from build123d import *

# Parameters (mm, degrees)
SKETCH001_W = 2773.187988
SKETCH001_H = 2729.466553
PAD_DEPTH   = 120


with BuildPart() as pad:
    # Sketch001 → Pad (new body)
    with BuildSketch(Plane.YZ):
        with Locations((0.000122, 6.245971)):
            Rectangle(SKETCH001_W, SKETCH001_H)
    extrude(amount=PAD_DEPTH)


with BuildPart() as cut:
    # Sketch → Revolution (revolve)
    with BuildSketch(Plane.XY):
        with BuildLine():
            ThreePointArc((14.647409, -801.533556), (158.5, -831.799058), (302.352591, -801.533556))
            Line((302.352591, -801.533556), (303.267814, -801.130607))
            ThreePointArc((303.267814, -801.130607), (313.263433, -792.647113), (317, -780.080485))
            Line((317, -780.070485), (317, -780.080485))
            ThreePointArc((317, -780.070485), (305.284271, -751.786214), (277, -740.070485))
            Line((40, -740.070485), (277, -740.070485))
            ThreePointArc((40, -740.070485), (11.715729, -751.786214), (0, -780.070485))
            Line((0, -780.070485), (0, -780.080485))
            ThreePointArc((0, -780.080485), (3.736567, -792.647113), (13.732186, -801.130607))
            Line((13.732186, -801.130607), (14.647409, -801.533556))
        make_face()
    revolve(axis=Axis((0, 0, 0), (1, 0, 0)))

    # Cut: cut Pad
    add(pad.part, mode=Mode.SUBTRACT)


solid = cut.part
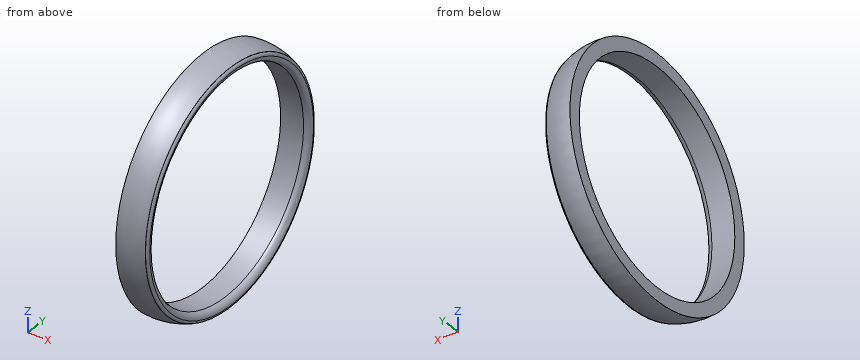
Read the model definition and answer for the solid it produces. Units are mm, in the model's axes. Coordinates: 2 decimals unless noted, no trailing zeros. Loops run counter-clockwise (first coordinate to the right, second up) from the corner with the lowest first, then second, coordinate; pieces in that order, holes last. Notation, with made-up numbers: (-2, 73) - (3, 73) arc R21 cw to (3, 100) - close; hole circle Ø3 at (21, -33). An arc over 180 degrees is marked (long way). Answer in a Markdown table with one row per item.
Q1. Straight lines are drawn through the part: line 1 along Y through (x, z) = (176, 0); line 2 along Y through (x, z) = (195, 0); line 3 along Z through (x, y) = (219, 0). For each, find the intervals that lie inside material, in ascending order. Write a range as [from, to].
Here are the results:
| item | result |
|---|---|
| line 1 | y = [-831.37, -740.07], [740.07, 831.37] |
| line 2 | y = [-829.93, -740.07], [740.07, 829.93] |
| line 3 | z = [-826.64, -740.07], [740.07, 826.64] |
Q2. Find section C-C on x = 240. Write down the section's boundary in (y, z).
Here are the results:
| item | result |
|---|---|
| outline | circle Ø1644.74 at (0, 0); hole circle Ø1480.14 at (0, 0) |
Q3. Given P1, Ø1, axis at x = 257, y = 122.5, coming from the +Z side; P2, Ø6, axis at x = 245, y = 312, coming from the +Z side; P3, Ø5, axis at x = 223.5, z = 585, coming from the -Y side, each flat-ended and moving along its own axis, determine where each tip first touches the part or whether it passes through.
Here are the results:
| item | result |
|---|---|
| P1 | stops at z = 808.88 |
| P2 | stops at z = 761.04 |
| P3 | stops at y = -585.48 |
